Model file for the job. Use its own axes, mm. Face numbers are marked on the shaded views. Give positions to 0.01 mm unless a question says otherwise; leave off trailing zeros. Order: outer loops, then holes, each group sorted by start corner. A loop starts at its lowest first (then second) coordinate and runs counter-clockwise, first axis right, second up. Notation, with made-up numbers: M 17.5,85 L 71.5,85 A17 cw 71.5,95 Z; hole C -10,58.5 d2. An arc over 180 degrees is marked long. Return JSON: item names as keys, results as strings. Group by question number.
1. Wall check: probe 1 along X at (y, z) = (89.25, 5.6); probe 2 along X at (y, z) = (90, 4.7); probe 3 along Y at (x, z) = (198, 5). Give the ranges that are in metal, low to high. Write a range as [from, to].
2. Slice it at B-B on y = 91.25. List the corners of the cut face in (x, z).
3. Slice it at D-D on y = 93.5. List the corners of the cut face in (x, z), then the cut area to 3 significant figures.
4. Slice it at C-C on x = 177.5. List the corners of the cut face in (y, z), then the cut area to 3 significant figures.
5. Slice it at A-A on z = 4.05. Give the number of separate pieces and of enclosed holes in the cut face, then the cut area to 3 significant figures.
6. Two-plate mould, pull along X, no slides. Class the marked faces 1, 2, 3 and 4: released by +X, released by -X, zero draft, split by the parting line, or undercut.
7. Pin check, flat tips, straight feed: pin 1 (2 mm diameter, centred on y = 87, z = 5.5, fed in from -X); pin 2 (1.5 mm diameter, centred on y = 92.5, z = 3, fed in from +X). Stop position of each tip, or through.
from build123d import *

# Parameters (mm, degrees)
DODANIE_WYCI_GNI_CIE1_DEPTH = 6
SZKIC2_R                    = 2.05
SZKIC2_R_2                  = 1.55
WYTNIJ_WYCI_GNI_CIE1_DEPTH  = 6


with BuildPart() as part:
    # Szkic1 → Dodanie-wyciągnięcie1 (new body)
    with BuildSketch(Plane.XY):
        with BuildLine():
            Line((148.389986738, 90.204311715), (148.389986738, 90.184311715))
            ThreePointArc((148.389986738, 90.184311715), (149.561559613, 87.35588459), (152.389986738, 86.184311715))
            Line((152.389986738, 86.184311715), (196.389986738, 86.184311715))
            ThreePointArc((196.389986738, 86.184311715), (199.218413863, 87.35588459), (200.389986738, 90.184311715))
            Line((200.389986738, 90.184311715), (200.389986738, 90.204311715))
            ThreePointArc((200.389986738, 90.204311715), (199.218413863, 93.032738839), (196.389986738, 94.204311715))
            Line((196.389986738, 94.204311715), (152.389986738, 94.204311715))
            ThreePointArc((152.389986738, 94.204311715), (149.561559613, 93.032738839), (148.389986738, 90.204311715))
        make_face()
    extrude(amount=DODANIE_WYCI_GNI_CIE1_DEPTH)

    # Szkic2 → Wytnij-wyciągnięcie1 (cut)
    with BuildSketch(Plane.XY.offset(6)):
        with Locations((196.389986738, 90.204311714)):
            Circle(SZKIC2_R)
        with Locations((178.389986738, 90.204311714)):
            Circle(SZKIC2_R_2)
        with Locations((152.389986738, 90.204311714)):
            Circle(SZKIC2_R_2)
    extrude(amount=-WYTNIJ_WYCI_GNI_CIE1_DEPTH, mode=Mode.SUBTRACT)


solid = part.part
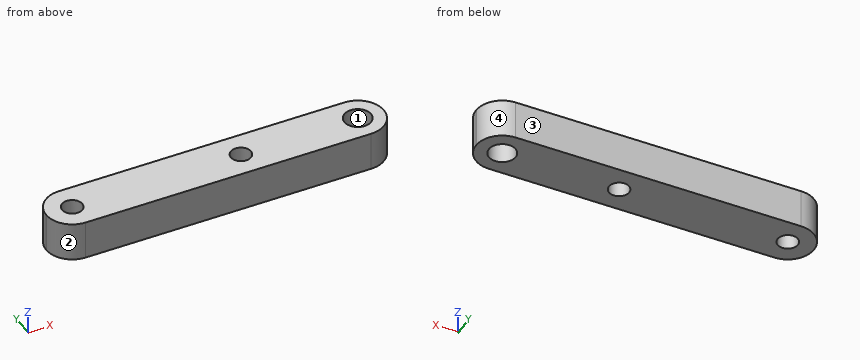
Result:
{
 "1": {"probe 1": "x = [148.5, 151.17], [153.61, 177.17], [179.61, 194.58], [198.2, 200.28]", "probe 2": "x = [148.39, 150.85], [153.93, 176.85], [179.93, 194.35], [198.43, 200.39]", "probe 3": "y = [86.52, 88.94], [91.47, 93.87]"},
 "2": {"outline": "M 148.53,0 L 151.25,0 L 151.25,6 L 148.53,6 Z; M 153.53,0 L 177.25,0 L 177.25,6 L 153.53,6 Z; M 179.53,0 L 194.63,0 L 194.63,6 L 179.53,6 Z; M 198.15,0 L 200.25,0 L 200.25,6 L 198.15,6 Z"},
 "3": {"outline": "M 150.12,0 L 198.66,0 L 198.66,6 L 150.12,6 Z", "area": "291 mm2"},
 "4": {"outline": "M 86.18,0 L 88.94,0 L 88.94,6 L 86.18,6 Z; M 91.47,0 L 94.2,0 L 94.2,6 L 91.47,6 Z", "area": "32.9 mm2"},
 "5": {"separate pieces": "1", "enclosed holes": "3", "area": "375 mm2"},
 "6": {"face 1": "undercut", "face 2": "released by -X", "face 3": "zero draft", "face 4": "released by +X"},
 "7": {"pin 1": "stops at x = 149.04", "pin 2": "stops at x = 200.08"}
}
